```python
from build123d import *

# Parameters (mm, degrees)
F1_DEPTH  = 2
F3_DEPTH  = 7
F4_SIZE   = 1.99999
F6_DEPTH  = 5
F8_DEPTH  = 5
F9_R      = 2.25
F10_DEPTH = 2
F11_R     = 4.5
F12_DEPTH = 2


# Not quite as in the source:
# - a fillet or chamfer is up to 0.001 mm smaller than in the source, because OpenCascade refuses the exact size


with BuildPart() as f1:
    # F0 (on Top) → F1 (new body)
    with BuildSketch(Plane.XY):
        Polygon((-28.5105540231, 5.458955369), (-0.5105540231, -1.9337359151), (22.9272134602, -36.1708849669), (33.0351494605, 13.7129257786), (41.5351494605, 16.0733799656), (41, 18.000454187), (-28, 7.3926912842), align=None)
    extrude(amount=F1_DEPTH)

    # F2 (on face) → F3 (join)
    with BuildSketch(Plane.XY.offset(2)):
        Polygon((-28.5105540231, 5.458955369), (-0.5105540231, -1.9337359151), (0, 0), (-28, 7.3926912842), align=None)
        Polygon((32.5, 15.64), (33.0351494605, 13.7129257786), (41.5351494605, 16.0733799656), (41, 18.000454187), align=None)
    extrude(amount=F3_DEPTH)

    # F4 (size 2 in the source; OpenCascade refuses exactly that, so slightly less here)
    f4_edges = [f1.edges().sort_by_distance(p)[0] for p in [
        (-14, 3.696346, 9),
        (36.75, 16.820227, 9),
    ]]
    chamfer(f4_edges, length=F4_SIZE)

    # F5 (on face) → F6 (join)
    with BuildSketch(Plane(origin=(0.8934695404, 3.3840378515, 3.5), x_dir=(0.9835734968, -0.125470625, -0.129770176), z_dir=(0.1805081059, 0.6836788893, 0.7071067812))):
        Polygon((-1.4274719357, -7.6460659082), (-0.9083912318, -4.8656783052), (-29.3760147392, 0.4490461714), (-29.8950954431, -2.3313414316), align=None)
    extrude(amount=F6_DEPTH)

    # F7 (on face) → F8 (join)
    with BuildSketch(Plane(origin=(-1.7892109036, 6.442951854, 6.6867708388), x_dir=(0.9819378198, 0.1312802997, 0.1362483066), z_dir=(-0.1892039063, 0.6813236249, 0.7071067812))):
        Polygon((43.5762937763, 8.105378656), (34.9199411754, 6.4055834869), (35.4649344018, 3.6301587657), (44.1212870028, 5.3299539348), align=None)
    extrude(amount=F8_DEPTH)

    # F9 (on face) → F10 (join)
    with BuildSketch(Plane(origin=(0, 0, 0), x_dir=(1, 0, 0), z_dir=(0, 0, -1))):
        with Locations((16.5175747303, -7.0523503236)):
            Circle(F9_R)
    extrude(amount=F10_DEPTH)

    # F11 (on face) → F12 (join)
    with BuildSketch(Plane(origin=(0, 0, -2), x_dir=(1, 0, 0), z_dir=(0, 0, -1))):
        with Locations((16.5175747303, -7.0523503236)):
            Circle(F11_R)
    extrude(amount=F12_DEPTH)


solid = f1.part
```
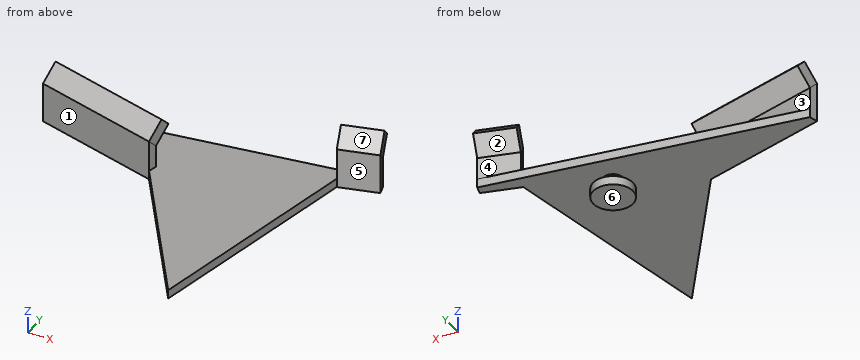
The model under review builds one solid part; all positions refer to its coordinate system, in mm. Face numbers are marked on the shaded views. A direction names the side the tool comes from. Give positions to 0.01 mm unless a question says otherwise; leave off trailing zeros. Write each loop counter-clockwise with the first axis right and the second up, starting at its lowest first coordinate (ties: lowest second). Pieces come first, ordered by that corner, then holes. Notation, with made-up numbers: M 57,37.5 L 106,37.5 A12 ccw 106,60.5 Z; hole C 66.5,36.25 d10. An arc over 180 degrees is marked long. Write item = value, one per line. Start each with the question number.
Q1. We need section D-D (y = -27). State the section outline as (x, z) points, plus the area to 3 significant figures.
Q2. Mouldability with a two-part tool opening along Z and no side actions: class the marked faces 4, 5, 6 and 7 as released by +Z, released by -Z, zero draft, split by the parting line, or undercut.
Q3. Clearance check with flat-ended pins moving along their axes: pin 1 (8 mm diameter, centred on y = -18, z = 6.5, fed in from -X); pin 2 (16.5 mm diameter, centred on x = 4, y = -9, fed in from +Z); pin 3 (8 mm diameter, centred on x = -4, z = 8, fed in from +Y). State where each tip first meets the part, or that it passes through.
Q4. We need section B-B (x = -2). State the section outline as (y, z) points.
Q5. Machinability: for the marked faces 1, 2 and 3, which of the approach directions +Z, -Z, +X, -X, +Y, -Y give a long, thin tool a straight path to every point of the face, cutting with its end or side? Answer none if there is none.
Q6. We need section A-A (z = 3.75). State the section outline as (x, y) points, plus the area to 3 significant figures.
Q7. We need section C-C (x = -14.5). State the section outline as (y, z) points, plus the area to 3 significant figures.
Q8. For line 1 (Z direction, x = 21, y = 11); line 2 (Z direction, x = -20.5, y = 8.5); line 3 (Y direction, x = -1, z = 8.5), list the stretches that pass through material, from the lowest coordinate up.
Result set:
q1.outline = M 16.65,0 L 24.79,0 L 24.79,2 L 16.65,2 Z
q1.area = 16.3 mm2
q2.face_4 = undercut
q2.face_5 = zero draft
q2.face_6 = released by -Z
q2.face_7 = released by +Z
q3.pin_1 = through
q3.pin_2 = 2
q3.pin_3 = 5.53
q4.outline = M -1.54,0 L 11.39,0 L 11.39,2 L 0.53,2 L 0.53,7 L 4.18,10.54 L 2.12,12.54 L -1.54,9 Z
q5.face_1 = +Z, -Z, -X, -Y
q5.face_2 = -X, +Y
q5.face_3 = +X, +Y
q6.outline = M -28.51,5.46 L -0.51,-1.93 L 0,0 L -28,7.39 Z; M 32.5,15.64 L 33.04,13.71 L 41.54,16.07 L 41,18 Z
q6.area = 75.6 mm2
q7.outline = M 1.76,0 L 9.47,0 L 9.47,2 L 3.83,2 L 3.83,7 L 7.49,10.54 L 5.42,12.54 L 1.76,9 Z
q7.area = 42.5 mm2
q8.line_1 = 0 to 2
q8.line_2 = 0 to 2, 9.99 to 11.09
q8.line_3 = -1.8 to 1.82
